from build123d import *

# Parameters (mm, degrees)
BASE_FLANGE1_DEPTH              = 31.75
FILLET1_R                       = 2.54
F_25_0_1495_DIAMETER_HOLE1_D    = 3.7973
SKETCH10_R                      = 5.715
CUT_EXTRUDE1_DEPTH              = 56.168930099
F_9_32_0_28125_DIAMETER_HOLE1_D = 7.14375
F_3_32_0_09375_DIAMETER_HOLE1_D = 2.38125
F_32_0_116_DIAMETER_HOLE1_D     = 2.9464


# Sheet-metal steps are written as plain solids
with BuildPart() as part:
    # Sketch3 → Base-Flange1 (new, symmetric)
    with BuildSketch(Plane(origin=(0, 0, 0), x_dir=(-1, 0, 0), z_dir=(0, 1, 0))):
        with BuildLine():
            Line((-33.3375, 0), (30.1625, 0))
            ThreePointArc((30.1625, 0), (32.40756403, -0.92993597), (33.3375, -3.175))
            Line((33.3375, -3.175), (33.3375, -25.4))
            Line((33.3375, -25.4), (35.6235, -25.4))
            Line((35.6235, -25.4), (35.6235, -3.175))
            ThreePointArc((35.6235, -3.175), (34.024010132, 0.686510132), (30.1625, 2.286))
            Line((30.1625, 2.286), (-33.3375, 2.286))
            Line((-33.3375, 2.286), (-33.3375, 0))
        make_face()
    extrude(amount=BASE_FLANGE1_DEPTH, both=True)

    # Fillet1
    fillet1_edges = [part.edges().sort_by_distance(p)[0] for p in [
        (33.3375, 31.75, 1.143),
        (33.3375, -31.75, 1.143),
        (-34.4805, 31.75, -25.4),
        (-34.4805, -31.75, -25.4),
    ]]
    fillet(fillet1_edges, radius=FILLET1_R)

    # #25 (0.1495) Diameter Hole1 (through all)
    with Locations(Plane.XY.offset(2.286)):
        with Locations((-23.8125, 19.05), (26.9875, 19.05), (26.9875, -19.05), (-23.8125, -19.05)):
            Hole(F_25_0_1495_DIAMETER_HOLE1_D / 2)

    # Sketch10 → Cut-Extrude1 (cut, through all)
    with BuildSketch(Plane.XY.offset(2.286)):
        Circle(SKETCH10_R)
    extrude(amount=-CUT_EXTRUDE1_DEPTH, mode=Mode.SUBTRACT)

    # 9/32 (0.28125) Diameter Hole1 (through all)
    with Locations(Plane.XY.offset(2.286)):
        with Locations((25.4, 0)):
            Hole(F_9_32_0_28125_DIAMETER_HOLE1_D / 2)

    # 3/32 (0.09375) Diameter Hole1 (through all)
    with Locations(Plane.XY.offset(2.286)):
        with Locations((0, 8.5), (0, -8.5)):
            Hole(F_3_32_0_09375_DIAMETER_HOLE1_D / 2)

    # #32 (0.116) Diameter Hole1 (through all)
    with Locations(Plane.XY.offset(2.286)):
        with Locations((15.057884182, 5.027499276), (15.057884182, -5.027499276)):
            Hole(F_32_0_116_DIAMETER_HOLE1_D / 2)


solid = part.part
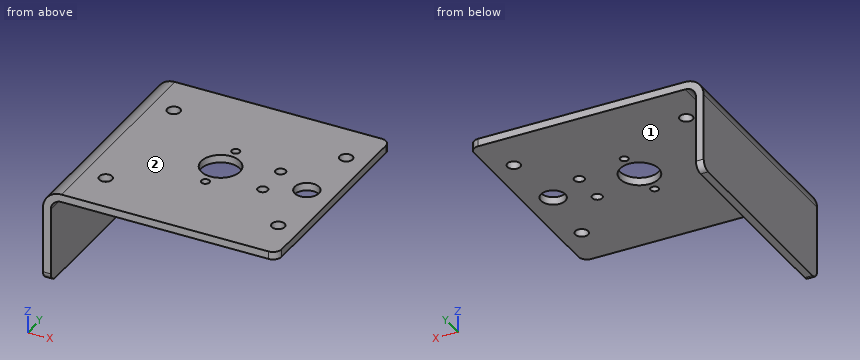
Design review of the part built by this model. Coordinates are the model's own, in mm. Face numbers are marked on the shaded views. A direction names the side the tool comes from. Coordinates: 2 decimals unless noted, no trailing zeros. Order: outer loops, then holes, each group sorted by start corner. A loop starts at its lowest first (then second) coordinate and runs counter-clockwise, first axis right, second up. Notation, with made-up numbers: (7.25, 50.25) - (46.25, 50.25) arc R21 cw to (46.25, 56.25) - close; hole circle Ø4 at (-3, 26). An arc over 180 degrees is marked (long way). Put each result on its own line as item: value.
1) Take a section at D-D, the plane z = -17.5. Give the boundary of the cut face in (x, y).
Response values:
outline: (-35.62, -31.75) - (-33.34, -31.75) - (-33.34, 31.75) - (-35.62, 31.75) - close
2) Wall thickness on L1, parallel to Y at x = 0, z = 0.8 (3 decimals); L2, parallel to Z at x = -19, y = 26.5; L3, parallel to X at y = 27, z = -4: over which ranges is each line inside the solid? List them lowest first. Write a range as from..to.
Response values:
L1: y = -31.75..-9.691, -7.309..-5.715, 5.715..7.309, 9.691..31.75
L2: z = 0..2.29
L3: x = -35.62..-33.34
3) Insertion check: P1, Ø11, axis at y = 8.5, z = -17, coming from the +X side; P2, Ø8, axis at x = 25.4, y = 0, coming from the -Z side; P3, Ø2.5, axis at x = 15.06, y = -5.03, coming from the -Z side; P4, Ø3, axis at x = 0, y = 8.5, coming from the +Z side. Each pin has a flat end and moves straight along its axis. Give the tip position at first contact, or say it passes through.
Response values:
P1: stops at x = -33.34
P2: stops at z = 0
P3: passes through
P4: stops at z = 2.29
4) Tool access review of the marked faces 1 and 2: name each direction out of +Z, -Z, +X, -X, +Y, -Y from which nothing blocks a thin tool from reaching the whole face with its end or side.
Response values:
face 1: -Z, +X, +Y, -Y
face 2: +Z, +X, -X, +Y, -Y
5) Take a section at A-A, the plane x = 0. Give the boundary of the cut face in (y, z) (3 decimals), and give its area (3 significant figures).
Response values:
outline: (-31.75, 0) - (-9.691, 0) - (-9.691, 2.286) - (-31.75, 2.286) - close; (-7.309, 0) - (-5.715, 0) - (-5.715, 2.286) - (-7.309, 2.286) - close; (5.715, 0) - (7.309, 0) - (7.309, 2.286) - (5.715, 2.286) - close; (9.691, 0) - (31.75, 0) - (31.75, 2.286) - (9.691, 2.286) - close
area: 108 mm²
6) Take a section at C-C, the plane y = 2.5. Count the separate pieces of the cut face and the enclosed holes in it, and give its area (3 significant figures).
Response values:
separate pieces: 3
enclosed holes: 0
area: 176 mm²
